The model under review builds one solid part; all positions refer to its coordinate system, in mm. A direction names the side the tool comes from. Coordinates: 2 decimals unless noted, no trailing zeros. Loops run counter-clockwise (first coordinate to the right, second up) from the corner with the lowest first, then second, coordinate; pieces in that order, holes last. Notation, with made-up numbers: (77, 36.5) - (91, 36.5) arc R11 cw to (91, 56.5) - close; hole circle Ø4 at (52, 74). An arc over 180 degrees is marked (long way). Answer in a Markdown table with one row per item. Add a question column.
(1) We need section B-B on y = 4. Write out the cut boundary in (x, z).
(2) We need section A-A on y = -14.5. Write out the cut boundary in (x, z).
(3) Mouldability with a two-part tool opening along Y and no side actions: class faces 6 (the flat face through (13, -42, 17.838)), 7 (the flat face through (12.52, -51.82, 29.62)), 8 (the flat face through (12.522, -13.473, 24.206)), 9 (the flat face through (12.52, 53.12, -5.45)) as +Y half, -Y half, draft (parallel to the pull), parting line (faces both ways), or undercut.
(4) For line 1 along Z through (x, y) = (22.5, -54.5); line 2 along Z through (x, y) = (8, -33); line 3 along Z through (x, y) = (4.25, 50.5), list the stretches that pass through material, from the lowest coordinate up.
(5) For P1, Ø2, axis at x = 15.5, z = 3.5, coming from the -Y side; P2, Ø5.5, axis at x = 11, y = -21.5, coming from the -Z side; P3, Ø6.5, axis at x = 13.5, z = 25.5, coming from the -Y side, all flat-tipped, find the tip position at first contact; note any pin that passes through.
(6) Machinability: for faces 1 (the flat face through (12.52, 23.87, 2.71)), 2 (the flat face through (12.522, -51.78, -13.045)), 3 (the flat face through (12.52, 30.58, -15.98)), 4 (the flat face through (12.522, 45.56, 38.566)), 5 (the flat face through (12.52, 47.03, 25.68)), which of the approach directions +Z, -Z, +X, -X, +Y, -Y give a long, thin tool a straight path to every point of the face, cutting with its end or side? Answer none if there is none.
(7) We need section C-C on z = 53.5. Write out the cut boundary in (x, y).
from build123d import *

# Parameters (mm, degrees)
F1_DEPTH = 25.4


with BuildPart() as f1:
    # F0 (on Right) → F1 (new body)
    with BuildSketch(Plane.YZ):
        with BuildLine():
            ThreePointArc((18.855748, -1.416255), (18.895578, -0.708625), (18.908861, 0))
            ThreePointArc((18.908861, 0), (18.838486, 1.629863), (18.627886, 3.247594))
            ThreePointArc((18.627886, 3.247594), (17.094445, 8.082386), (14.330997, 12.335621))
            ThreePointArc((14.330997, 12.335621), (11.890608, 14.702328), (9.065882, 16.593818))
            ThreePointArc((9.065882, 16.593818), (-0.204608, 18.907754), (-9.422852, 16.393745))
            ThreePointArc((-9.422852, 16.393745), (-13.441603, 13.299185), (-16.493181, 9.247701))
            ThreePointArc((-16.493181, 9.247701), (-17.741605, 6.540678), (-18.549073, 3.67109))
            ThreePointArc((-18.549073, 3.67109), (-18.89422, -0.743959), (-18.202995, -5.118202))
            ThreePointArc((-18.202995, -5.118202), (-15.727938, -10.496522), (-11.710979, -14.845807))
            ThreePointArc((-11.710979, -14.845807), (-0.498769, -18.902281), (10.911764, -15.442746))
            ThreePointArc((10.911764, -15.442746), (13.834686, -12.889782), (16.17484, -9.793853))
            ThreePointArc((16.17484, -9.793853), (18.009208, -5.763111), (18.855748, -1.416255))
        make_face()
        with BuildLine():
            ThreePointArc((14.330997, 12.335621), (17.094445, 8.082386), (18.627886, 3.247594))
            Line((18.627886, 3.247594), (35.620206, 10.771734))
            Line((35.620206, 10.771734), (27.777187, 13.626359))
            Line((27.777187, 13.626359), (43.256562, 15.996829))
            Line((43.256562, 15.996829), (33.913499, 19.397426))
            Line((33.913499, 19.397426), (52.177158, 23.806515))
            Line((52.177158, 23.806515), (41.743724, 27.603975))
            Line((41.743724, 27.603975), (54.702936, 41.603265))
            Line((54.702936, 41.603265), (36.156493, 35.442327))
            Line((36.156493, 35.442327), (34.117385, 41.580712))
            Line((34.117385, 41.580712), (28.336922, 25.699019))
            Line((28.336922, 25.699019), (25.773159, 33.416785))
            Line((25.773159, 33.416785), (21.026523, 20.375509))
            Line((21.026523, 20.375509), (20.743884, 29.954885))
            Line((20.743884, 29.954885), (14.330997, 12.335621))
        make_face()
        with BuildLine():
            Line((28.741808, 6.718539), (18.855748, -1.416255))
            ThreePointArc((18.855748, -1.416255), (18.009208, -5.763111), (16.17484, -9.793853))
            Line((16.17484, -9.793853), (24.926406, -16.084017))
            Line((24.926406, -16.084017), (27.179874, -9.892665))
            Line((27.179874, -9.892665), (34.0759, -22.243811))
            Line((34.0759, -22.243811), (37.2388, -13.553815))
            Line((37.2388, -13.553815), (47.768776, -25.455565))
            Line((47.768776, -25.455565), (46.683991, -16.991583))
            Line((46.683991, -16.991583), (62.231524, -18.952553))
            Line((62.231524, -18.952553), (48.904825, -7.480339))
            Line((48.904825, -7.480339), (57.452464, -3.363933))
            Line((57.452464, -3.363933), (39.655712, -0.83815))
            Line((39.655712, -0.83815), (44.267129, 3.420753))
            Line((44.267129, 3.420753), (28.815001, 3.107546))
            Line((28.815001, 3.107546), (28.741808, 6.718539))
        make_face()
        with BuildLine():
            ThreePointArc((-9.422852, 16.393745), (-0.204608, 18.907754), (9.065882, 16.593818))
            Line((9.065882, 16.593818), (17.664263, 31.343678))
            Line((17.664263, 31.343678), (9.065882, 27.197644))
            Line((9.065882, 27.197644), (20.08703, 44.887555))
            Line((20.08703, 44.887555), (9.065882, 39.573293))
            Line((9.065882, 39.573293), (16.843367, 59.706657))
            Line((16.843367, 59.706657), (9.065882, 55.690415))
            Line((9.065882, 55.690415), (0, 73.246568))
            Line((0, 73.246568), (-9.422852, 55.211404))
            Line((-9.422852, 55.211404), (-15.973218, 62.022142))
            Line((-15.973218, 62.022142), (-9.422852, 41.58793))
            Line((-9.422852, 41.58793), (-18.851278, 46.768438))
            Line((-18.851278, 46.768438), (-9.422852, 27.215003))
            Line((-9.422852, 27.215003), (-17.412247, 31.802535))
            Line((-17.412247, 31.802535), (-9.422852, 16.393745))
        make_face()
        with BuildLine():
            Line((16.388254, -33.097774), (10.911764, -15.442746))
            ThreePointArc((10.911764, -15.442746), (-0.498769, -18.902281), (-11.710979, -14.845807))
            Line((-11.710979, -14.845807), (-17.786112, -33.097774))
            Line((-17.786112, -33.097774), (16.388254, -33.097774))
        make_face()
        with BuildLine():
            ThreePointArc((-16.493181, 9.247701), (-13.441603, 13.299185), (-9.422852, 16.393745))
            Line((-9.422852, 16.393745), (-22.304947, 29.787894))
            Line((-22.304947, 29.787894), (-22.304947, 21.441529))
            Line((-22.304947, 21.441529), (-29.826717, 35.176635))
            Line((-29.826717, 35.176635), (-29.826717, 25.233954))
            Line((-29.826717, 25.233954), (-40.216446, 40.888183))
            Line((-40.216446, 40.888183), (-40.216446, 29.785154))
            Line((-40.216446, 29.785154), (-57.803787, 37.174791))
            Line((-57.803787, 37.174791), (-45.671143, 21.854))
            Line((-45.671143, 21.854), (-50.741921, 17.838414))
            Line((-50.741921, 17.838414), (-33.840977, 17.838414))
            Line((-33.840977, 17.838414), (-40.216446, 12.789634))
            Line((-40.216446, 12.789634), (-26.33821, 12.789634))
            Line((-26.33821, 12.789634), (-35.24321, 9.247701))
            Line((-35.24321, 9.247701), (-16.493181, 9.247701))
        make_face()
        with BuildLine():
            Line((-24.710589, -16.143639), (-18.202995, -5.118202))
            ThreePointArc((-18.202995, -5.118202), (-18.89422, -0.743959), (-18.549073, 3.67109))
            Line((-18.549073, 3.67109), (-28.924217, 6.588699))
            Line((-28.924217, 6.588699), (-28.924217, 0))
            Line((-28.924217, 0), (-39.628703, 9.247701))
            Line((-39.628703, 9.247701), (-39.628703, 0))
            Line((-39.628703, 0), (-53.594282, 7.582523))
            Line((-53.594282, 7.582523), (-49.680065, 0))
            Line((-49.680065, 0), (-64.960659, -3.474861))
            Line((-64.960659, -3.474861), (-48.51393, -9.697216))
            Line((-48.51393, -9.697216), (-55.138189, -16.488837))
            Line((-55.138189, -16.488837), (-37.550844, -12.775449))
            Line((-37.550844, -12.775449), (-40.427528, -18.354706))
            Line((-40.427528, -18.354706), (-26.014401, -12.775449))
            Line((-26.014401, -12.775449), (-24.710589, -16.143639))
        make_face()
    extrude(amount=F1_DEPTH)


solid = f1.part
Outcome:
| question | item | result |
|---|---|---|
| 1 | outline | (0, -33.1) - (25.4, -33.1) - (25.4, 65.5) - (0, 65.5) - close |
| 2 | outline | (0, -33.1) - (25.4, -33.1) - (25.4, -23.23) - (0, -23.23) - close; (0, -12.14) - (25.4, -12.14) - (25.4, 21.67) - (0, 21.67) - close; (0, 26.19) - (25.4, 26.19) - (25.4, 30.13) - (0, 30.13) - close; (0, 37.74) - (25.4, 37.74) - (25.4, 44.38) - (0, 44.38) - close; (0, 57.43) - (25.4, 57.43) - (25.4, 60.49) - (0, 60.49) - close |
| 3 | face 6 | draft |
| 3 | face 7 | -Y half |
| 3 | face 8 | undercut |
| 3 | face 9 | +Y half |
| 4 | line 1 | -16.35 to -15.83, -7.43 to -1.1, 33 to 35.79 |
| 4 | line 2 | -15.48 to 3.52, 9.25 to 10.14, 12.79 to 30.02 |
| 4 | line 3 | -17.47 to -8.85, -6.71 to -2.38, 23.4 to 24.42, 37.06 to 40.21 |
| 5 | P1 | y = -52 |
| 5 | P2 | z = -15.36 |
| 5 | P3 | y = -51.13 |
| 6 | face 1 | +X, -X |
| 6 | face 2 | +X, -X, -Y |
| 6 | face 3 | -Z, +X, -X |
| 6 | face 4 | +Z, +X, -X |
| 6 | face 5 | +X, -X, +Y |
| 7 | outline | (0, -13.24) - (25.4, -13.24) - (25.4, 14.45) - (0, 14.45) - close |
